Can you work these out from the drawing? Everything is in mm from the part's minimum corner. A direction names the side the tool comes from. Round coordinates to 2 decimals unless told otherwise and drop trailing zeros. Order: outer loops, then holes, each group sorted by start corner. A loop starts at its lowest first (then second) coordinate and runs counter-clockwise, first axis right, second up. Notation, with made-up numbers: (29.25, 19) -> (60.25, 19) arc R21 ccw to (60.25, 54) -> close; hole circle Ø3 at (18.5, 18.25). An arc over 180 degrees is marked (long way). One line per item, written item: value.
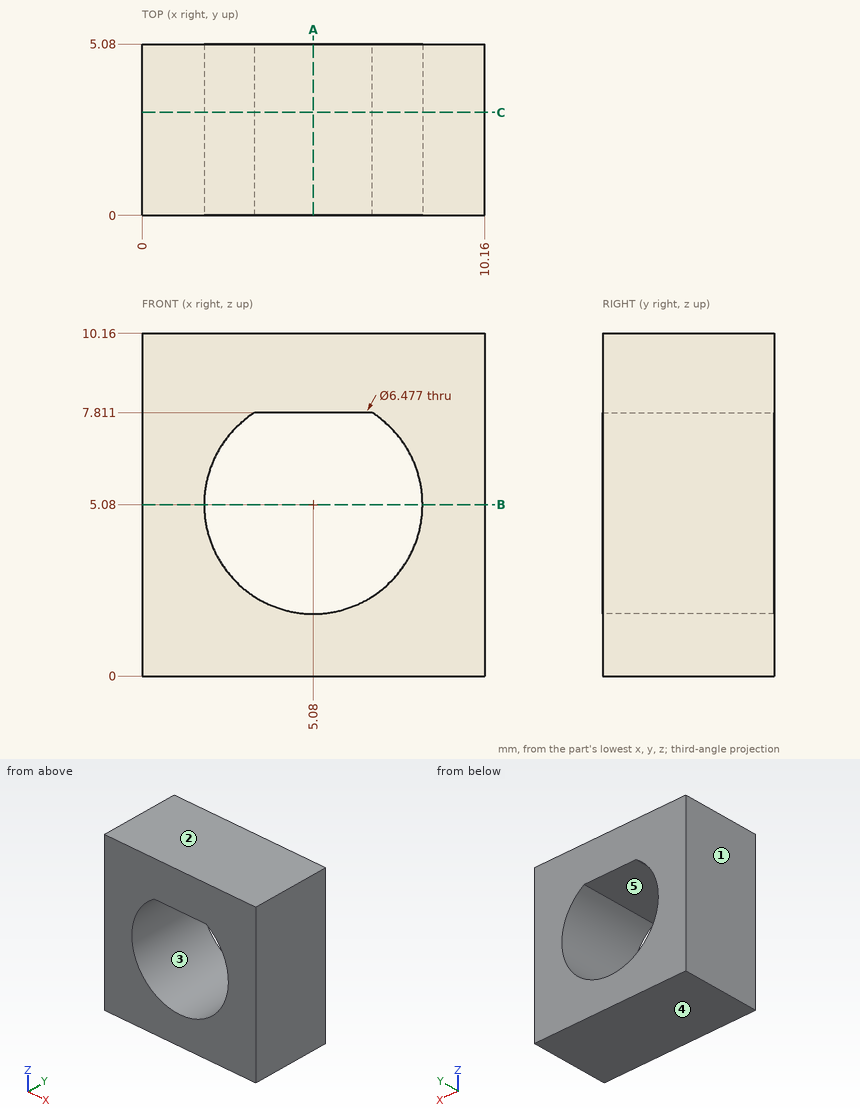
Q1. I want a section at C-C on y = 3.05. Write out the boundary of the cut face in (x, z).
Answers:
outline: (0, 0) -> (10.16, 0) -> (10.16, 10.16) -> (0, 10.16) -> close; hole (3.34, 7.81) arc R3.24 ccw (long way) to (6.82, 7.81) -> close
Q2. I need wall thicknesses on line 1 along Z through (x, y) = (5.08, 2.25); line 2 along X through (y, z) = (3.45, 5); line 3 along Z through (x, y) = (6.5, 0.8). Which ranges of each line are inside material? Lowest first, please.
Answers:
line 1: 0 to 1.84, 7.81 to 10.16
line 2: 0 to 1.84, 8.32 to 10.16
line 3: 0 to 2.17, 7.81 to 10.16
Q3. If we mould it in two halves opening along Z, with no side actions, what happens to the marked faces 1, 2 and 3? For each: pulls with the +Z half, pulls with the -Z half, needs draft (parallel to the pull), parting line crosses it, or undercut.
Answers:
face 1: needs draft
face 2: pulls with the +Z half
face 3: undercut
Q4. I want a section at B-B on z = 5.08. Write out the boundary of the cut face in (x, y).
Answers:
outline: (0, 0) -> (1.84, 0) -> (1.84, 5.08) -> (0, 5.08) -> close; (8.32, 0) -> (10.16, 0) -> (10.16, 5.08) -> (8.32, 5.08) -> close
Q5. Which directions (+Z, -Z, +X, -X, +Y, -Y) give clear straight access to the entire face, cutting with the end or side of a thin tool? Please do the marked faces 4 and 5.
Answers:
face 4: -Z, +X, -X, +Y, -Y
face 5: +Y, -Y
Q6. For P1, Ø1, axis at x = 8, z = 2, coming from the -Y side, with a flat end and sliding along its axis, tell me the tip position at first contact or that it passes through.
Answers:
P1: y = 0
Q7. I want a section at A-A on x = 5.08. Write out the boundary of the cut face in (y, z).
Answers:
outline: (0, 0) -> (5.08, 0) -> (5.08, 1.84) -> (0, 1.84) -> close; (0, 7.81) -> (5.08, 7.81) -> (5.08, 10.16) -> (0, 10.16) -> close
